```python
from build123d import *

# Parameters (mm, degrees)
SKETCH1_R           = 12.573
BOSS_EXTRUDE1_DEPTH = 76.2
SKETCH2_R           = 21.0185
BOSS_EXTRUDE2_DEPTH = 6.35
FILLET1_R           = 0.762


with BuildPart() as part:
    # Sketch1 → Boss-Extrude1 (new body)
    with BuildSketch(Plane.XY):
        Circle(SKETCH1_R)
    extrude(amount=-BOSS_EXTRUDE1_DEPTH)

    # Sketch2 → Boss-Extrude2 (add)
    with BuildSketch(Plane.XY):
        Circle(SKETCH2_R)
    extrude(amount=BOSS_EXTRUDE2_DEPTH)

    # Fillet1
    fillet1_edges = [part.edges().sort_by_distance(p)[0] for p in [
        (-21.0185, 0, 0),
        (-21.0185, 0, 6.35),
    ]]
    fillet(fillet1_edges, radius=FILLET1_R)


solid = part.part
```
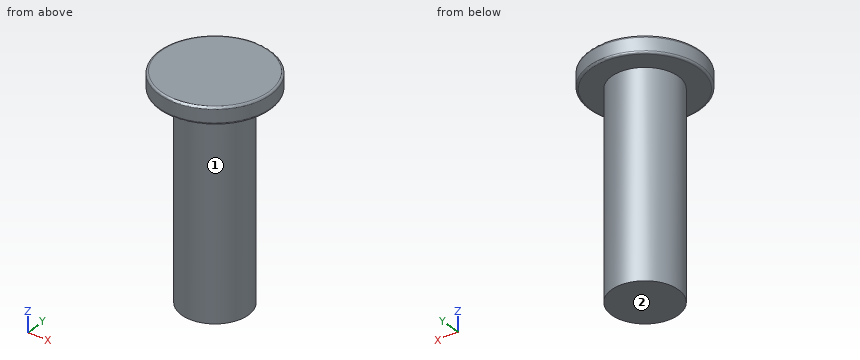
CAD build for the part. Positions are in the model's coordinates, mm. Face numbers are marked on the shaded views. A direction names the side the tool comes from. Round coordinates to 2 decimals unless told otherwise and drop trailing zeros. Write each loop counter-clockwise with the first axis right and the second up, starting at its lowest first coordinate (ties: lowest second). Pieces come first, ordered by that corner, then holes. Notation, with made-up numbers: M 3,38.5 L 39,38.5 A22 ccw 39,53.5 Z; hole C 84,-21.5 d5. An arc over 180 degrees is marked long. One line per question, with ' | ' between items.
1. Pin check, flat tips, straight feed: pin 1 Ø12 at (y, z) = (-2.5, -62.5) entering from +X; pin 2 Ø3 at (y, z) = (-13, -2.5) entering from +X; pin 3 Ø6 at (x, z) = (10.5, -59) entering from -Y. Stop position of each tip, or through.
Working result:
pin 1: x = 12.57 | pin 2: x = 5.08 | pin 3: y = -10.09
2. Which spindle directions (+Z, -Z, +X, -X, +Y, -Y) get a long thin tool onto all of the face, cutting with end or side? Do the marked faces 1 and 2. Say none if no direction does.
Working result:
face 1: -Z | face 2: -Z, +X, -X, +Y, -Y
3. Probe L1, parallel to Z at x = 2, y = -16; L2, parallel to X at y = 11.5, z = -24.5; L3, parallel to X at y = -7, z = -59.5. List the from-to ranges inside material, lowest first. Write a range as from..to.
Working result:
L1: 0..6.35 | L2: -5.08..5.08 | L3: -10.44..10.44
4. Cut at C-C on z = -31. Write the cut outline in (x, y).
Working result:
outline: C 0,0 d25.15
5. Cut at A-A on y = 0. Write the cut outline in (x, z).
Working result:
outline: M -21.02,0.76 A0.76 ccw -20.26,0 L -12.57,0 L -12.57,-76.2 L 12.57,-76.2 L 12.57,0 L 20.26,0 A0.76 ccw 21.02,0.76 L 21.02,5.59 A0.76 ccw 20.26,6.35 L -20.26,6.35 A0.76 ccw -21.02,5.59 Z
